Verification items for the finished model (mm, model axes). A direction names the side the tool comes from. Give positions to 0.01 mm unless a question says otherwise; leave off trailing zeros. Loops run counter-clockwise (first coordinate to the right, second up) from the corner with the lowest first, then second, coordinate; pieces in that order, holes last. Notation, with made-up numbers: M 54.25,17 L 65.25,17 A25 cw 65.25,38 Z; hole C 78,-34.5 d10. An arc over 180 degrees is marked long. Answer in a Markdown table with one row per item.
```python
from build123d import *

# Parameters (mm, degrees)
SKETCH1_R           = 5
BOSS_EXTRUDE1_DEPTH = 1
SKETCH2_R           = 4
BOSS_EXTRUDE4_DEPTH = 4
SKETCH5_R           = 2.5
CUT_EXTRUDE4_DEPTH  = 4
SKETCH6_R           = 1.25
CUT_EXTRUDE5_DEPTH  = 4
SKETCH7_R           = 1.5
CUT_EXTRUDE6_DEPTH  = 10


with BuildPart() as part:
    # Sketch1 → Boss-Extrude1 (new body)
    with BuildSketch(Plane(origin=(0, 0, 0), x_dir=(1, 0, 0), z_dir=(0, 1, 0))):
        with Locations(Location((0, 0, 0), (0, 0, 270))):
            Circle(SKETCH1_R)
    extrude(amount=BOSS_EXTRUDE1_DEPTH)

    # Sketch2 → Boss-Extrude4 (add)
    with BuildSketch(Plane(origin=(0, 1, 0), x_dir=(1, 0, 0), z_dir=(0, 1, 0))):
        with Locations(Location((0, 0, 0), (0, 0, 270))):
            Circle(SKETCH2_R)
    extrude(amount=BOSS_EXTRUDE4_DEPTH)

    # Sketch5 → Cut-Extrude4 (cut)
    with BuildSketch(Plane(origin=(0, 5, 0), x_dir=(1, 0, 0), z_dir=(0, 1, 0))):
        with Locations(Location((0, 0, 0), (0, 0, 270))):
            Circle(SKETCH5_R)
    extrude(amount=-CUT_EXTRUDE4_DEPTH, mode=Mode.SUBTRACT)

    # Sketch6 → Cut-Extrude5 (cut)
    with BuildSketch(Plane(origin=(0, 1, 0), x_dir=(1, 0, 0), z_dir=(0, 1, 0))):
        with Locations(Location((0, 0, 0), (0, 0, 270))):
            Circle(SKETCH6_R)
    extrude(amount=-CUT_EXTRUDE5_DEPTH, mode=Mode.SUBTRACT)

    # Sketch7 → Cut-Extrude6 (cut)
    with BuildSketch(Plane.XZ):
        with Locations(Location((0, 0, 0), (0, 0, 270))):
            Circle(SKETCH7_R)
    extrude(amount=-CUT_EXTRUDE6_DEPTH, mode=Mode.SUBTRACT)


solid = part.part
```
Item 1: Scan lines: L1, parallel to X at y = 1.5, z = 0; L2, parallel to X at y = 0.55, z = 0; L3, parallel to Y at x = -3.75, z = 3. Record each from-to range of solid material in increasing order. Write a range as [from, to].
Reported:
| item | result |
|---|---|
| L1 | x = [-4, -2.5], [2.5, 4] |
| L2 | x = [-5, -1.5], [1.5, 5] |
| L3 | y = [0, 1] |
Item 2: Go/stop test with flat-tipped pins: pin 1 (5 mm diameter, centred on x = -2.5, z = 3, fed in from -Y); pin 2 (2 mm diameter, centred on x = 2.5, y = 2.5, fed in from -Z); pin 3 (3.5 mm diameter, centred on x = 0, z = 0, fed in from +Y); pin 4 (1 mm diameter, centred on y = 2, z = -3, fed in from +X). Record where each tip stops, or that it passes through.
Reported:
| item | result |
|---|---|
| pin 1 | stops at y = 0 |
| pin 2 | stops at z = -3.71 |
| pin 3 | stops at y = 1 |
| pin 4 | stops at x = 3.12 |
Item 3: Sectioned sample at D-D (z = -1.75). Record the cut outline in (x, y).
Reported:
| item | result |
|---|---|
| outline | M -4.68,0 L 4.68,0 L 4.68,1 L 3.6,1 L 3.6,5 L 1.79,5 L 1.79,1 L -1.79,1 L -1.79,5 L -3.6,5 L -3.6,1 L -4.68,1 Z |
Item 4: Release check for a two-part mould opening along X. For faces 3 (the cylindrical face through (-2.44, 3.03, -0.54)), 4 (the cylindrical face through (-3.905, 2.972, -0.867)), 5 (the cylindrical face through (0.45, 0.49, -1.43)), 6 (the flat face through (2, 5, 2)) record: released by +X, released by -X, zero draft, split by the parting line, or undercut.
Reported:
| item | result |
|---|---|
| face 3 | undercut |
| face 4 | split by the parting line |
| face 5 | undercut |
| face 6 | zero draft |
Item 5: Sectioned sample at A-A (x = 0). Record the cut outline in (y, z), and give its area (3 significant figures).
Reported:
| item | result |
|---|---|
| outline | M 0,-5 L 1,-5 L 1,-4 L 5,-4 L 5,-2.5 L 1,-2.5 L 1,-1.5 L 0,-1.5 Z; M 0,1.5 L 1,1.5 L 1,2.5 L 5,2.5 L 5,4 L 1,4 L 1,5 L 0,5 Z |
| area | 19.0 mm^2 |
Item 6: Tool access check on faces 1 (the flat face through (-2, 1, 0)), 2 (the flat face through (1.2, 0, -1.2)). Record the directions out of +Z, -Z, +X, -X, +Y, -Y that give a thin tool (end or side, any length) a straight path to the whole face; none if there is none.
Reported:
| item | result |
|---|---|
| face 1 | +Y |
| face 2 | +Z, -Z, +X, -X, -Y |
Item 7: Sectioned sample at C-C (y = 3.95). Record the cut outline in (x, z).
Reported:
| item | result |
|---|---|
| outline | C 0,0 d8; hole C 0,0 d5 |
Item 8: Sectioned sample at B-B (z = 0). Record the cut outline in (x, y).
Reported:
| item | result |
|---|---|
| outline | M -5,0 L -1.5,0 L -1.5,1 L -2.5,1 L -2.5,5 L -4,5 L -4,1 L -5,1 Z; M 1.5,0 L 5,0 L 5,1 L 4,1 L 4,5 L 2.5,5 L 2.5,1 L 1.5,1 Z |
